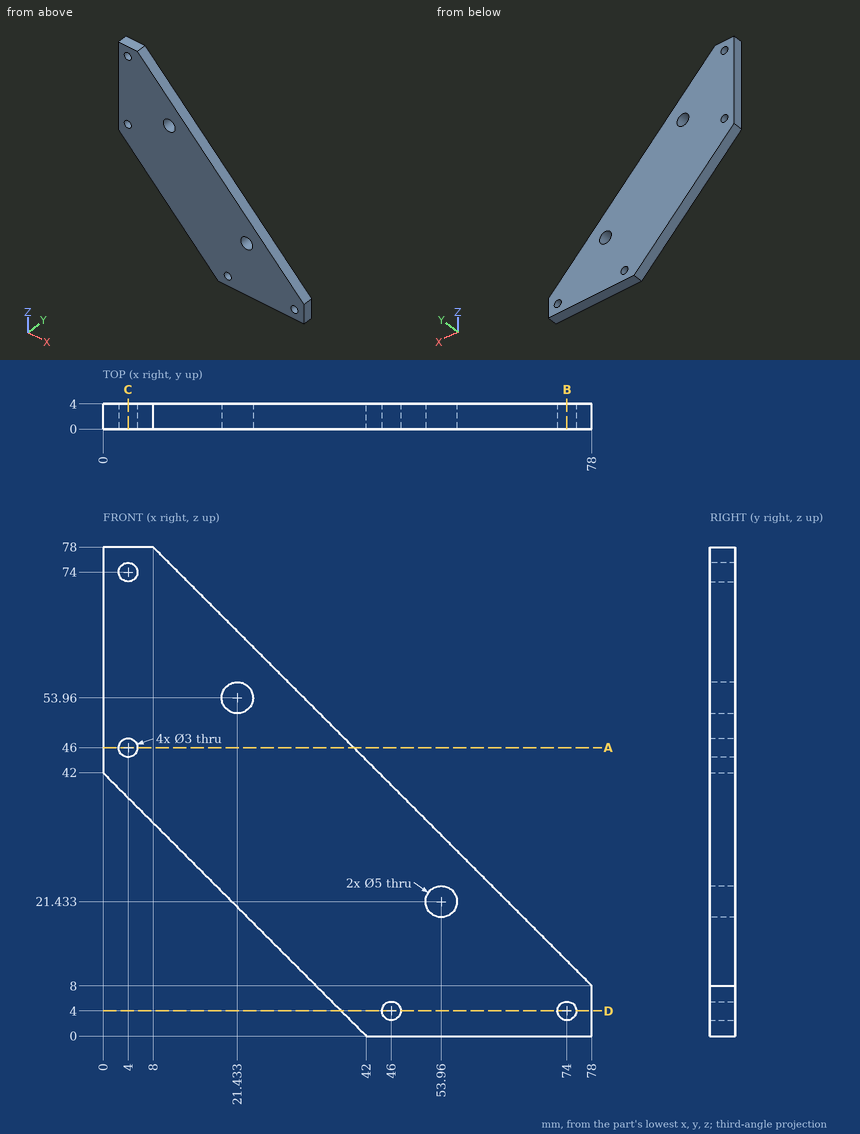
Part print with two shaded views. Sizes in mm from the minimum x, y, z corner. Round coordinates to 2 decimals unless told otherwise and drop trailing zeros. Order: outer loops, then holes, each group sorted by start corner. A loop starts at its lowest first (then second) coordinate and runs counter-clockwise, first axis right, second up.
(1) Band-saw the part on C-C (x = 4). List the corners of the cut face in (y, z).
(2) Band-saw the part on A-A (z = 46). List the corners of the cut face in (x, y), then the cut area to 3 significant figures.
(3) Drill centre lines: line 1 (X direction, y = 0.2, z = 5); line 2 (X direction, y = 2.3, z = 4); line 3 (X direction, y = 2.6, z = 74). Where is each one in solid material? Low to high.
(4) Band-saw the part on B-B (x = 74). List the corners of the cut face in (y, z), then the cut area to 3 significant figures.
(5) Band-saw the part on D-D (z = 4). List the corners of the cut face in (x, y).
(6) Pin check, flat tips, straight feed: pin 1 (1.5 mm diameter, centred on y = 1.5, z = 64.5, fed in from +X); pin 2 (1.8 mm diameter, centred on x = 74, z = 4, fed in from +Y); pin 3 (1 mm diameter, centred on y = 1, z = 37, fed in from -X); pin 4 (1.5 mm diameter, centred on y = 1, z = 63, fed in from +X). Stop position of each tip, or through.
Verdict:
1. outline: (0, 38) - (4, 38) - (4, 44.5) - (0, 44.5) - close; (0, 47.5) - (4, 47.5) - (4, 72.5) - (0, 72.5) - close; (0, 75.5) - (4, 75.5) - (4, 78) - (0, 78) - close
2. outline: (0, 0) - (2.5, 0) - (2.5, 4) - (0, 4) - close; (5.5, 0) - (40, 0) - (40, 4) - (5.5, 4) - close
2. area: 148 mm2
3. line 1: x = 37 to 44.88, 47.12 to 72.88, 75.12 to 78
3. line 2: x = 38 to 44.5, 47.5 to 72.5, 75.5 to 78
3. line 3: x = 0 to 2.5, 5.5 to 12
4. outline: (0, 0) - (4, 0) - (4, 2.5) - (0, 2.5) - close; (0, 5.5) - (4, 5.5) - (4, 12) - (0, 12) - close
4. area: 36.0 mm2
5. outline: (38, 0) - (44.5, 0) - (44.5, 4) - (38, 4) - close; (47.5, 0) - (72.5, 0) - (72.5, 4) - (47.5, 4) - close; (75.5, 0) - (78, 0) - (78, 4) - (75.5, 4) - close
6. pin 1: stops at x = 22.25
6. pin 2: passes through
6. pin 3: stops at x = 4.5
6. pin 4: stops at x = 23.75
